Part model, mm, in its own coordinate system. A direction names the side the tool comes from. Give positions to 0.01 mm unless a question says otherwise; leave off trailing zeros. Answer in a Markdown table with one row per item.
from build123d import *

# Parameters (mm, degrees)
SHELL1_T           = -6.35
SKETCH4_W          = 81.861054952
SKETCH4_H          = 81.861054952
CUT_EXTRUDE1_DEPTH = 117.570504586


with BuildPart() as part:
    # Sketch1 → Loft1 section 0
    with BuildSketch(Plane.XY):
        with BuildLine():
            Line((-44.45, 44.45), (44.45, 44.45))
            Line((44.45, 44.45), (44.45, -44.45))
            Line((44.45, -44.45), (-44.45, -44.45))
            Line((-44.45, -44.45), (-44.45, 44.45))
        make_face()
    # Sketch2 → Loft1 section 1
    with BuildSketch(Plane.XY.offset(50.8)):
        with BuildLine():
            Line((-76.2, 76.2), (76.2, 76.2))
            Line((76.2, 76.2), (76.2, -76.2))
            Line((76.2, -76.2), (-76.2, -76.2))
            Line((-76.2, -76.2), (-76.2, 76.2))
        make_face()
    loft()

    # Shell1
    shell1_openings = [part.faces().sort_by_distance(p)[0] for p in [
        (0, 0, 50.8),
    ]]
    offset(amount=SHELL1_T, openings=shell1_openings, kind=Kind.INTERSECTION)

    # Sketch4 → Cut-Extrude1 (cut, through all)
    with BuildSketch(Plane.XY.offset(6.35)):
        Rectangle(SKETCH4_W, SKETCH4_H)
    extrude(amount=-CUT_EXTRUDE1_DEPTH, mode=Mode.SUBTRACT)


solid = part.part
(1) Pull direction X, two halves, no side cores. Call faces 3 (the face through (40.931, -1, 3)), 4 (the face through (3, -42, 0)): +X half, -X half, draft (parallel to the pull), parting line (faces both ways), or undercut.
Recorded:
| item | result |
|---|---|
| face 3 | undercut |
| face 4 | draft |
(2) Drill centre lines: line 1 along Y through (x, z) = (-40.5, 31) (3 decimals); line 2 along X through (y, z) = (27, 19) (3 decimals); line 3 along Y through (x, z) = (12, 17.5). Where is each one in solid material? Low to high.
Recorded:
| item | result |
|---|---|
| line 1 | y = -63.825 to -56.337, 56.337 to 63.825 |
| line 2 | x = -56.325 to -48.837, 48.837 to 56.325 |
| line 3 | y = -55.39 to -47.9, 47.9 to 55.39 |
(3) Which spindle directions (+Z, -Z, +X, -X, +Y, -Y) get a long thin tool onto all of the face, cutting with end or side? Do faces 1 (the face through (-6, 74, 50.8)), 2 (the face through (-1, -40.931, 3)). Say none if no direction does.
Recorded:
| item | result |
|---|---|
| face 1 | +Z, +X, -X, +Y, -Y |
| face 2 | +Z, -Z |
(4) Pin check, flat tips, straight feed: pin 1 Ø5 at (x, z) = (32.5, 8.5) entering from +Y (3 decimals); pin 2 Ø5 at (y, z) = (32, 23) entering from -X; pin 3 Ø3 at (y, z) = (5.5, 3) entering from -X. Stop position of each tip, or through.
Recorded:
| item | result |
|---|---|
| pin 1 | stops at y = 51.325 |
| pin 2 | stops at x = -60.39 |
| pin 3 | stops at x = -47.26 |
